Could you check a few things on this model? Use its own coordinates, in mm. A direction names the side the tool comes from. Round coordinates to 2 decimals unless told otherwise and drop trailing zeros. Write each loop counter-clockwise with the first axis right and the second up, starting at its lowest first coordinate (ties: lowest second). Pieces come first, ordered by that corner, then holes. Notation, with made-up numbers: (-17, 47.5) - (17, 47.5) arc R9 cw to (17, 53.5) - close; hole circle Ø10 at (35, 71). An arc over 180 degrees is marked (long way). Put each result on its own line as item: value.
Autodesk Inventor part; units mm, degrees
ref_plane "YZ Plane" through (0, 0, 0) normal (1, 0, 0) x (0, 1, 0)
ref_plane "XZ Plane" through (0, 0, 0) normal (0, 1, 0) x (-1, 0, 0)
ref_plane "XY Plane" through (0, 0, 0) normal (0, 0, 1) x (1, 0, 0)
sketch "Sketch1" plane through (0, 0, 0) normal (0, 0, 1) x (1, 0, 0)
  line L0 (0, 0) -> (42, 0)
  line L1 (42, 0) -> (42, 6)
  line L2 (42, 6) -> (0, 6)
  line L3 (0, 6) -> (0, 0)
  line L4 (6, 6) -> (14, 6)
  line L5 (14, 6) -> (14, 10)
  line L6 (14, 10) -> (6, 10)
  line L7 (6, 10) -> (6, 6)
  line L8 (28, 6) -> (36, 6)
  line L9 (36, 6) -> (36, 10)
  line L10 (36, 10) -> (28, 10)
  line L11 (28, 10) -> (28, 6)
  dimension "d0" = 42
  dimension "d1" = 6
  dimension "d2" = 4
  dimension "d3" = 8
  dimension "d4" = 8
  dimension "d5" = 6
  dimension "d6" = 6
extrude "Extrusion1" add sketch "Sketch1" along normal blind 38.1
sketch "Sketch2" plane through (0, 0, 0) normal (0, -1, 0) x (1, 0, 0)
  line L0 (0, 0) -> (42, 0)
  line L1 (0, 0) -> (0, 38.1)
  point P0 (21, 19.05)
  dimension "d9" = 19.05
  dimension "d10" = 21
hole "Hole1" at (21, 0, 19.05) direction (0, 1, 0) diameter 3.175 end through all
sketch "Sketch3" plane through (0, 0, 38.1) normal (0, 0, 1) x (1, 0, 0)
  line L0 (0, 0) -> (42, 0)
  line L1 (0, 6) -> (1, 6)
  line L2 (1, 6) -> (1, 0)
  line L3 (1, 0) -> (0, 0)
  line L4 (0, 0) -> (0, 6)
  line L5 (42, 6) -> (41, 6)
  line L6 (41, 6) -> (41, 0)
  line L7 (41, 0) -> (42, 0)
  line L8 (42, 0) -> (42, 6)
  dimension "d18" = 1
  dimension "d19" = 1
extrude "Extrusion2" cut sketch "Sketch3" against normal blind 50.8
equation "\"d4\" = d3"
equation "\"d6\" = d5"
properties part number "Slider" material "PET Plastic"
(1) Imagine slicing it at A-A, the plane x = 21. List the corners of the cut face in (y, z) for me, then the cut area to 3 significant figures.
Values found:
outline: (0, 0) - (6, 0) - (6, 17.46) - (0, 17.46) - close; (0, 20.64) - (6, 20.64) - (6, 38.1) - (0, 38.1) - close
area: 210 mm^2
(2) Imagine slicing it at C-C, the plane y = 8.75. List the corners of the cut face in (x, z) for me.
Values found:
outline: (6, 0) - (14, 0) - (14, 38.1) - (6, 38.1) - close; (28, 0) - (36, 0) - (36, 38.1) - (28, 38.1) - close
(3) Imagine slicing it at D-D, the plane z = 34.5. List the corners of the cut face in (x, y) for me.
Values found:
outline: (1, 0) - (41, 0) - (41, 6) - (36, 6) - (36, 10) - (28, 10) - (28, 6) - (14, 6) - (14, 10) - (6, 10) - (6, 6) - (1, 6) - close
(4) For faces 1 (the face through (36, 8, 19)), 2 (the face through (28, 8, 19)), 3 (the face through (4, 6, 19)), which set-ups out of +Z, -Z, +X, -X, +Y, -Y let a thin tool reach every point of the face, with its end or its side?
Values found:
face 1: +Z, -Z, +X, +Y
face 2: +Z, -Z, +Y
face 3: +Z, -Z, -X, +Y
(5) Imagine slicing it at B-B, the plane z = 19.05. List the corners of the cut face in (x, y) for me.
Values found:
outline: (1, 0) - (19.41, 0) - (19.41, 6) - (14, 6) - (14, 10) - (6, 10) - (6, 6) - (1, 6) - close; (22.59, 0) - (41, 0) - (41, 6) - (36, 6) - (36, 10) - (28, 10) - (28, 6) - (22.59, 6) - close
(6) Please list where these lines run through material, in increasing order: probe 1 along Z at (x, y) = (21, 3.35); probe 2 along X at (y, z) = (3.95, 19.05); probe 3 along X at (y, z) = (6.5, 35). Write a range as from..to.
Values found:
probe 1: z = 0..17.46, 20.64..38.1
probe 2: x = 1..19.41, 22.59..41
probe 3: x = 6..14, 28..36
(7) I'm going to push flat-ended pins straight in: pin 1 (2 mm diameter, centred on y = 8.5, z = 10, fed in from -X); pin 2 (1.2 mm diameter, centred on y = 8.5, z = 13, fed in from +X); pin 3 (1.5 mm diameter, centred on x = 2.5, z = 10.5, fed in from +Y); pin 4 (2.5 mm diameter, centred on x = 21, z = 19.05, fed in from +Y). Where does each tip first touch, or does it pass through?
Values found:
pin 1: stops at x = 6
pin 2: stops at x = 36
pin 3: stops at y = 6
pin 4: passes through
